from build123d import *

# Parameters (mm, degrees)
F0_W     = 20
F0_H     = 30
F1_DEPTH = 35


with BuildPart() as f1:
    # F0 (on Top) → F1 (new body)
    with BuildSketch(Plane.XY):
        Polygon((-33.5, -7), (-30.5, -7), (-30.5, 27), (-33.5, 27), (-53.929, 27), (-53.929, -7), align=None)
        with Locations((-41.929, 10)):
            Rectangle(F0_W, F0_H, mode=Mode.SUBTRACT)
        Polygon((30.5, 30.5), (30.5, 27), (33.5, 27), (33.5, 33.5), (-33.5, 33.5), (-33.5, 27), (-30.5, 27), (-30.5, 30.5), align=None)
        Polygon((30.5, 27), (30.5, -7), (33.5, -7), (53.929, -7), (53.929, 27), (33.5, 27), align=None)
        with Locations((41.929, 10)):
            Rectangle(F0_W, F0_H, mode=Mode.SUBTRACT)
        Polygon((30.5, -7), (30.5, -30.5), (-30.5, -30.5), (-30.5, -7), (-33.5, -7), (-33.5, -33.5), (33.5, -33.5), (33.5, -7), align=None)
    extrude(amount=F1_DEPTH)


solid = f1.part
Read the model definition and answer for the solid it produces. Units are mm, in the model's axes. A direction names the side the tool comes from. Round coordinates to 2 decimals unless told otherwise and drop trailing zeros. Loops run counter-clockwise (first coordinate to the right, second up) from the corner with the lowest first, then second, coordinate; pieces in that order, holes last. Notation, with made-up numbers: (51, 86.25) - (66, 86.25) arc R10 ccw to (66, 105.25) - close; hole circle Ø11 at (65, 18.25). An arc over 180 degrees is marked (long way). One line per question, with ' | ' between items. Start each with the question number.
Q1. For faces 1 (the flat face through (-33.5, 30, 17)), 2 (the flat face through (-44, -7, 17)), 3 (the flat face through (51.929, 10, 17)), 4 (the flat face through (33.5, 30, 17)), determine the directions among +Z, -Z, +X, -X, +Y, -Y from which every point of the face is accessible in a straight line to the end or side of a thin tool.
Q2. Section D-D on x = 36.5 is taken. Give the vertices of the cut face in (y, z).
Q3. Flat-ended cylindrical pins translate along their axes: pin 1 (3 mm diameter, centred on y = 31.5, z = 12, fed in from +X); pin 2 (6 mm diameter, centred on x = -45.5, z = 12.5, fed in from -Y); pin 3 (6 mm diameter, centred on x = 47, z = 12, fed in from +Y). Find the tip coordinate at first contact, or state that the pin passes through.
Q4. For a pull along Y with two mould halves and no side action, classify faces 5 (the flat face through (-31.929, 10, 17)), 6 (the flat face through (33.5, -20, 17)), 7 (the flat face through (30.5, 0, 17)), 8 (the flat face through (-44, 27, 17)) as +Y half, -Y half, draft (parallel to the pull), parting line (faces both ways), or undercut.
Q5. Section C-C on z = 13 is taken. Give the vertices of the cut face in (x, y).
Q6. Find the intervals of material crossed by L1, parallel to X at y = -1, z = 7; L2, parallel to Y at x = -1, z = 26, in increasing order.
Q7. Section A-A on x = -15.5 is taken. Give the vertices of the cut face in (y, z).
Q8. Section B-B on y = 5 is taken. Give the vertices of the cut face in (x, z).
Established:
1) face 1: +Z, -Z, -X, +Y | face 2: +Z, -Z, -X, -Y | face 3: +Z, -Z | face 4: +Z, -Z, +X, +Y
2) outline: (-7, 0) - (-5, 0) - (-5, 35) - (-7, 35) - close; (25, 0) - (27, 0) - (27, 35) - (25, 35) - close
3) pin 1: x = 33.5 | pin 2: y = -7 | pin 3: y = 27
4) face 5: undercut | face 6: draft | face 7: undercut | face 8: +Y half
5) outline: (-53.93, -7) - (-33.5, -7) - (-33.5, -33.5) - (33.5, -33.5) - (33.5, -7) - (53.93, -7) - (53.93, 27) - (33.5, 27) - (33.5, 33.5) - (-33.5, 33.5) - (-33.5, 27) - (-53.93, 27) - close; hole (-51.93, -5) - (-31.93, -5) - (-31.93, 25) - (-51.93, 25) - close; hole (-30.5, -30.5) - (30.5, -30.5) - (30.5, 30.5) - (-30.5, 30.5) - close; hole (31.93, -5) - (51.93, -5) - (51.93, 25) - (31.93, 25) - close
6) L1: -53.93 to -51.93, -31.93 to -30.5, 30.5 to 31.93, 51.93 to 53.93 | L2: -33.5 to -30.5, 30.5 to 33.5
7) outline: (-33.5, 0) - (-30.5, 0) - (-30.5, 35) - (-33.5, 35) - close; (30.5, 0) - (33.5, 0) - (33.5, 35) - (30.5, 35) - close
8) outline: (-53.93, 0) - (-51.93, 0) - (-51.93, 35) - (-53.93, 35) - close; (-31.93, 0) - (-30.5, 0) - (-30.5, 35) - (-31.93, 35) - close; (30.5, 0) - (31.93, 0) - (31.93, 35) - (30.5, 35) - close; (51.93, 0) - (53.93, 0) - (53.93, 35) - (51.93, 35) - close
